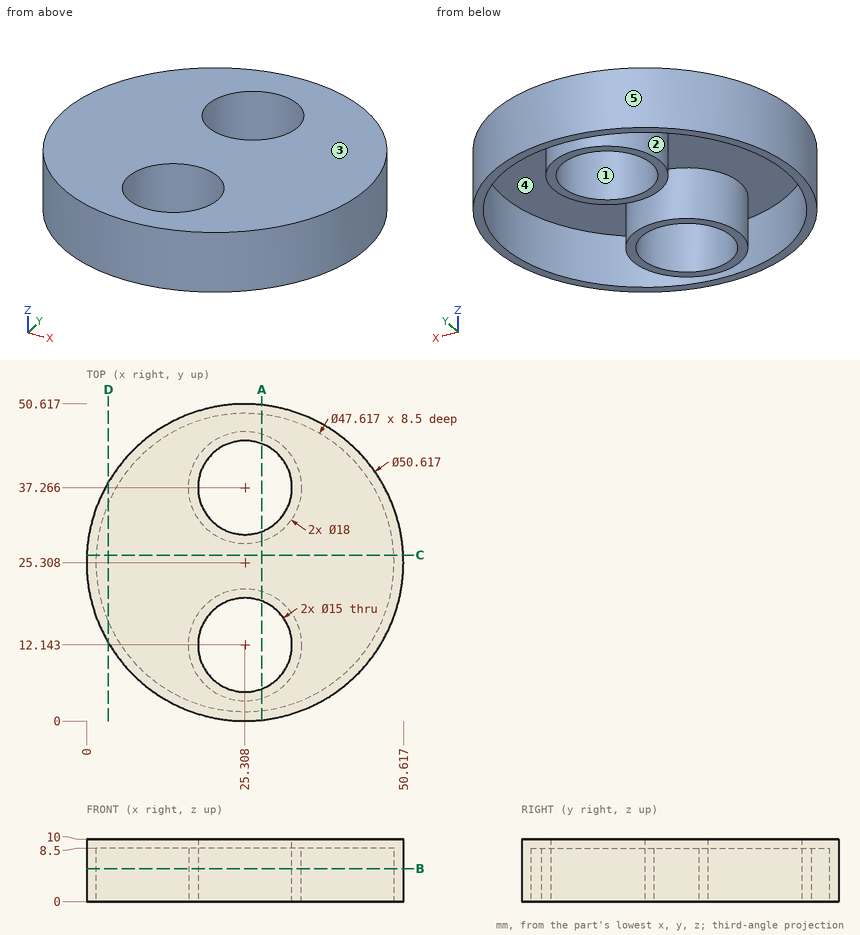
Study the drawing (mm; zero at the part's minimum x, y, z) and answer. A direction names the side the tool comes from. Coordinates: 2 decimals unless noted, no trailing zeros. Loops run counter-clockwise (first coordinate to the right, second up) from the corner with the lowest first, then second, coordinate; pieces in that order, holes last. Notation, with made-up numbers: M 17.5,29 L 22.5,29 A7 cw 22.5,34 Z; hole C -9.75,-37 d7. An arc over 180 degrees is marked long. Answer in a Markdown table with one row per item. Add a question column.
1. Find section D-D, the plane x = 3.5. Write down the section's boundary in (y, z).
2. Find section B-B, the plane z = 5.25. Write down the section's boundary in (x, y).
3. The mould has two halves that part along X. Classify the marked faces 3, 4 and 5: pulls with the +X half, pulls with the -X half, needs draft (parallel to the pull), parting line crosses it, or undercut.
4. Find section A-A, the plane x = 28. Write down the section's boundary in (y, z) (1 decimal), then the cut area to 3 significant figures.
5. A tool of negligible diameter and unlimited length cuts with its end or side. For the marked faces 1 and 2, from which of +Z, -Z, +X, -X, +Y, -Y can it reach the whole face along a straight path? Write none if from no direction.
6. Consider L1, parallel to Y at x = 26.5, z = 4.5 (1 decimal); L2, parallel to X at y = 16, z = 4.5 (1 decimal); L3, parallel to X at y = 18.5, z = 6.5 (1 decimal). Determine where each line is inside the solid, lowest interval first.
7. Flat-ended cylindrical pins translate along their axes: P1, Ø1, axis at x = 42, z = 8.5, coming from the -Y side; P2, Ø5, axis at y = 44, z = 6.5, coming from the -X side. Find the tip coordinate at first contact, or state that the pin passes through.
8. Find section C-C, the plane y = 26.5. Write down the section's boundary in (x, z).
Reported:
| question | item | result |
|---|---|---|
| 1 | outline | M 12.47,0 L 15.76,0 L 15.76,8.5 L 34.86,8.5 L 34.86,0 L 38.15,0 L 38.15,10 L 12.47,10 Z |
| 2 | outline | C 25.31,25.31 d50.62; C 25.31,12.14 d18; C 25.31,37.27 d18; hole C 25.31,25.31 d47.62; hole C 25.31,12.14 d15; hole C 25.31,37.27 d15 |
| 3 | face 3 | needs draft |
| 3 | face 4 | undercut |
| 3 | face 5 | parting line crosses it |
| 4 | outline | M 0.1,0 L 1.7,0 L 1.7,8.5 L 3.6,8.5 L 3.6,0 L 5.1,0 L 5.1,10 L 0.1,10 Z; M 19.1,0 L 20.7,0 L 20.7,8.5 L 28.7,8.5 L 28.7,0 L 30.3,0 L 30.3,10 L 19.1,10 Z; M 44.3,0 L 45.9,0 L 45.9,8.5 L 49,8.5 L 49,0 L 50.5,0 L 50.5,10 L 44.3,10 Z |
| 4 | area | 113 mm^2 |
| 5 | face 1 | +Z, -Z |
| 5 | face 2 | -Z |
| 6 | L1 | y = 0 to 1.5, 3.2 to 4.7, 19.5 to 21.1, 28.3 to 29.9, 44.7 to 46.2, 49.1 to 50.6 |
| 6 | L2 | x = 1.8 to 3.4, 17.2 to 18.9, 31.7 to 33.4, 47.2 to 48.8 |
| 6 | L3 | x = 0.9 to 2.5, 18.9 to 21.3, 29.3 to 31.7, 48.1 to 49.7 |
| 7 | P1 | stops at y = 5.86 |
| 7 | P2 | stops at x = 5.86 |
| 8 | outline | M 0.03,0 L 1.53,0 L 1.53,8.5 L 49.09,8.5 L 49.09,0 L 50.59,0 L 50.59,10 L 0.03,10 Z |
